Build history of the part. All positions in model axes, mm. A direction names the side the tool comes from. Give positions to 0.01 mm unless a question says otherwise; leave off trailing zeros. Loops run counter-clockwise (first coordinate to the right, second up) from the corner with the lowest first, then second, coordinate; pieces in that order, holes last. Notation, with made-up numbers: (82.5, 37.25) -> (93.5, 37.25) arc R9 cw to (93.5, 41.25) -> close; hole circle Ø8 at (-33.5, -12.5). An arc over 180 degrees is marked (long way). One line per question, with ' | ' between items. Start each with the question number.
(1) 3-axis set-ups, long thin cutter, end or side, ignore diameter. For faces 3 (the face through (29.053, -5.402, -5.204)), 4 (the face through (12.13, -1.48, -72.39)): which of +Z, -Z, +X, -X, +Y, -Y reach the whole face in a straight line?
(2) Mould opens along Z. For faces 1 (the face through (30.997, -3.45, -39.092)), 2 (the face through (22, 0, -53)) say: pulls with the +Z half, pulls with the -Z half, needs draft (parallel to the pull), parting line crosses it, or undercut.
(3) Slice it at A-A, the plane y = -5.5. Give the number of separate pieces and of enclosed holes in the cut face, then the cut area to 3 significant figures.
(4) Flat gauge pins, fed straight in: pin 1 Ø6 at (x, z) = (16.44, -48.51) entering from +Y; pin 2 Ø3 at (x, z) = (22.5, -28) entering from +Y; pin 3 Ø1.8 at (x, z) = (30.5, -6) entering from +Y. Where does each tip first touch, or does it go through?
(5) Drill centre lines: L1, parallel to X at y = -3.25, z = -68.5; L2, parallel to Z at x = 24, y = -4.75; L3, parallel to Z at x = 24.5, y = -4. Where is each one in solid material? Low to high. Write a range as from..to.
(6) Slice it at B-B, the plane z = -38.1. Write the cut outline in (x, y), then the cut area to 3 significant figures.
```python
from build123d import *

# Parameters (mm, degrees)
BOSS_EXTRUDE2_DEPTH = 6.35
SKETCH7_R           = 5
CUT_EXTRUDE1_DEPTH  = 74.422
SKETCH22_R          = 1.7907
CUT_EXTRUDE2_DEPTH  = 74.422
SKETCH21_R          = 1.25
CUT_EXTRUDE3_DEPTH  = 74.422


with BuildPart() as part:
    # Sketch3 → Boss-Extrude2 (new body)
    with BuildSketch(Plane(origin=(0, 0, 0), x_dir=(1, 0, 0), z_dir=(0, 1, 0))):
        with BuildLine():
            Line((30.988, 73.406), (51.21275, 4.064))
            ThreePointArc((51.21275, 4.064), (50.70475, 1.27), (48.16475, 0))
            Line((48.16475, 0), (22.076833333, 0))
            Line((22.076833333, 0), (0, 75.692))
            Line((0, 75.692), (27.94, 75.692))
            ThreePointArc((27.94, 75.692), (29.845, 75.057), (30.988, 73.406))
        make_face()
    extrude(amount=-BOSS_EXTRUDE2_DEPTH)

    # Sketch7 → Cut-Extrude1 (cut)
    with BuildSketch(Plane(origin=(0, 0, 0), x_dir=(0, 0, -1), z_dir=(1, 0, 0))):
        with Locations((6.857884732, 2.831164756)):
            Circle(SKETCH7_R)
        with Locations((17.279310179, 3.596191936)):
            Circle(SKETCH7_R)
        with Locations((27.691863994, 4.053898332)):
            Circle(SKETCH7_R)
        with Locations((38.1, 4.20625)):
            Circle(SKETCH7_R)
        with Locations((48.508136006, 4.053898332)):
            Circle(SKETCH7_R)
        with Locations((58.920689821, 3.596191936)):
            Circle(SKETCH7_R)
        with Locations((69.342115268, 2.831164756)):
            Circle(SKETCH7_R)
    extrude(amount=CUT_EXTRUDE1_DEPTH, mode=Mode.SUBTRACT)

    # Sketch22 → Cut-Extrude2 (cut)
    with BuildSketch(Plane(origin=(0, 0, 0), x_dir=(1, 0, 0), z_dir=(0, 1, 0))):
        with Locations(Location((9.789583333, 69.342, 0), (0, 0, 270))):
            Circle(SKETCH22_R)
        with Locations(Location((16.439386687, 48.514, 0), (0, 0, 270))):
            Circle(SKETCH22_R)
        with Locations(Location((23.08919004, 27.686, 0), (0, 0, 270))):
            Circle(SKETCH22_R)
        with Locations(Location((29.738993393, 6.858, 0), (0, 0, 270))):
            Circle(SKETCH22_R)
    extrude(amount=-CUT_EXTRUDE2_DEPTH, mode=Mode.SUBTRACT)

    # Sketch21 → Cut-Extrude3 (cut)
    with BuildSketch(Plane(origin=(0, 0, 0), x_dir=(1, 0, 0), z_dir=(0, 1, 0))):
        with Locations(Location((19.473333333, 69.342, 0), (0, 0, 270))):
            Circle(SKETCH21_R)
        with Locations(Location((23.568118499, 58.928, 0), (0, 0, 270))):
            Circle(SKETCH21_R)
        with Locations(Location((27.662903665, 48.514, 0), (0, 0, 270))):
            Circle(SKETCH21_R)
        with Locations(Location((31.757688831, 38.1, 0), (0, 0, 270))):
            Circle(SKETCH21_R)
        with Locations(Location((35.852473996, 27.686, 0), (0, 0, 270))):
            Circle(SKETCH21_R)
        with Locations(Location((39.947259162, 17.272, 0), (0, 0, 270))):
            Circle(SKETCH21_R)
        with Locations(Location((44.042044328, 6.858, 0), (0, 0, 270))):
            Circle(SKETCH21_R)
    extrude(amount=-CUT_EXTRUDE3_DEPTH, mode=Mode.SUBTRACT)

    # Sketch24 → Cut-Revolve1 (revolve, cut)
    with BuildSketch(Plane(origin=(9.789583333, 0, 0), x_dir=(0, 0, -1), z_dir=(1, 0, 0)), mode=Mode.PRIVATE) as cut_revolve1_sk:
        Polygon((69.342, 1.594870185), (69.342, -2.168835243), (69.342, -4.480235243), (71.1454, -4.480235243), (73.184910088, -2.215129815), (73.184910088, 1.594870185), align=None)
    revolve(cut_revolve1_sk.sketch.rotate(Axis((9.789583333, 1.594870185, -69.342), (0, -1, 0)), 180), axis=Axis((9.789583333, 1.594870185, -69.342), (0, -1, 0)), mode=Mode.SUBTRACT)

    # Sketch26 → Cut-Revolve2 (revolve, cut)
    with BuildSketch(Plane(origin=(16.439386687, 0, 0), x_dir=(0, 0, -1), z_dir=(1, 0, 0)), mode=Mode.PRIVATE) as cut_revolve2_sk:
        Polygon((48.514, -0.946098229), (48.514, -3.257498229), (50.3174, -3.257498229), (52.356910088, -0.992392801), (52.356910088, 3.057918479), (48.514, 3.057918479), align=None)
    revolve(cut_revolve2_sk.sketch.rotate(Axis((16.439386687, 3.057918479, -48.514), (0, -1, 0)), 180), axis=Axis((16.439386687, 3.057918479, -48.514), (0, -1, 0)), mode=Mode.SUBTRACT)

    # Sketch28 → Cut-Revolve3 (revolve, cut)
    with BuildSketch(Plane(origin=(23.08919004, 0, 0), x_dir=(0, 0, -1), z_dir=(1, 0, 0))):
        Polygon((27.686, 3.057918479), (27.686, -0.946098229), (27.686, -3.257498229), (25.8826, -3.257498229), (23.843089912, -0.992392801), (23.843089912, 3.057918479), align=None)
    revolve(axis=Axis((23.08919004, 3.057918479, -27.686), (0, -1, 0)), mode=Mode.SUBTRACT)

    # Sketch29 → Cut-Revolve4 (revolve, cut)
    with BuildSketch(Plane(origin=(29.738993393, 0, 0), x_dir=(0, 0, -1), z_dir=(1, 0, 0))):
        Polygon((3.015089912, 1.594870185), (6.858, 1.594870185), (6.858, -2.168835243), (6.858, -4.480235243), (5.0546, -4.480235243), (3.015089912, -2.215129815), align=None)
    revolve(axis=Axis((29.738993393, 1.594870185, -6.858), (0, -1, 0)), mode=Mode.SUBTRACT)


solid = part.part
```
Final values:
1) face 3: +Y, -Y | face 4: +Y
2) face 1: undercut | face 2: needs draft
3) separate pieces: 1 | enclosed holes: 11 | area: 2,220 mm2
4) pin 1: y = -1.92 | pin 2: y = -2.85 | pin 3: y = -4.21
5) L1: 2.1..7, 12.58..18.55, 20.4..32.42 | L2: -75.69..-60.1, -57.75..-29.23, -26.14..0 | L3: -75.69..-59.76, -58.09..-28.79, -26.58..0
6) outline: (10.96, -6.35) -> (30.51, -6.35) -> (30.51, -0.79) -> (10.96, -0.79) -> close; (33.01, -6.35) -> (41.29, -6.35) -> (41.29, -0.79) -> (33.01, -0.79) -> close | area: 155 mm2
